```python
from build123d import *

# Parameters (mm, degrees)
F1_DEPTH = 25.4
F2_R     = 3.3782
F3_DEPTH = 25.4
F4_R     = 3.3782
F5_DEPTH = 25.4


with BuildPart() as f1:
    # F0 (on Right) → F1 (new body)
    with BuildSketch(Plane.YZ):
        Polygon((0, 38.1), (0, 0), (38.1, 0), (38.1, 3.175), (3.175, 3.175), (3.175, 38.1), align=None)
    extrude(amount=F1_DEPTH)

    # F2 (on face) → F3 (cut)
    with BuildSketch(Plane.XZ):
        with Locations((12.7, 19.05)):
            Circle(F2_R)
    extrude(amount=-F3_DEPTH, mode=Mode.SUBTRACT)

    # F4 (on face) → F5 (cut)
    with BuildSketch(Plane(origin=(0, 0, 0), x_dir=(1, 0, 0), z_dir=(0, 0, -1))):
        with Locations((12.7, -19.05)):
            Circle(F4_R)
    extrude(amount=-F5_DEPTH, mode=Mode.SUBTRACT)


solid = f1.part
```
Could you check a few things on this model? Use its own coordinates, in mm. A direction names the side the tool comes from. Coordinates: 2 decimals unless noted, no trailing zeros. Order: outer loops, then holes, each group sorted by start corner. A loop starts at its lowest first (then second) coordinate and runs counter-clockwise, first axis right, second up. Notation, with made-up numbers: M 6,65 L 62,65 A29 ccw 62,85 Z; hole C 52.5,60 d1. An arc over 180 degrees is marked long. Use a Markdown table: item, result. Add a question column.
Q1. I'm going to push a flat-ended pin straight in: pin 1 (1 mm diameter, centred on x = 5, z = 19.5, fed in from +Y) (3 decimals). Where does the tip first touch, or does it pass through?
Q2. I want a section at A-A on y = 19.05. List the corners of the cut face in (x, z) for me (3 decimals), then the cut area to 3 significant figures.
Q3. If I drill on L1, parallel to X at y = 19.05, z = 2; L2, parallel to Y at x = 12.7, z = 0.95; L3, parallel to Z at x = 17.5, y = 8 (3 decimals), over which ranges is the centre line in solid material (lowest first)?
Q4. I want a section at B-B on x = 12.7. List the corners of the cut face in (y, z) for me (3 decimals).
Q5. I want a section at D-D on x = 15.25. List the corners of the cut face in (y, z) for me (3 decimals).
Q6. Which directions (+Z, -Z, +X, -X, +Y, -Y) give clear straight access to the entire face, cutting with the end or side of a thin tool? Please do faces 1 (the flat face through (13, 2, 38.1)), 2 (the flat face through (13, 25, 3.175)).
Q7. We'd pull the mould along X, two halves only. Please class faces 3 (the cylindrical face through (12.26, 15.7, 1.57)), 4 (the cylindrical face through (11.97, 1.57, 15.75)), 5 (the flat face through (25.4, 2, 11)), 6 (the flat face through (13, 38.1, 2)): pulls with the +X half, pulls with the -X half, needs draft (parallel to the pull), parting line crosses it, or undercut.
Checked values:
| question | item | result |
|---|---|---|
| 1 | pin 1 | y = 3.175 |
| 2 | outline | M 0,0 L 9.322,0 L 9.322,3.175 L 0,3.175 Z; M 16.078,0 L 25.4,0 L 25.4,3.175 L 16.078,3.175 Z |
| 2 | area | 59.2 mm² |
| 3 | L1 | 0 to 9.32, 16.08 to 25.4 |
| 3 | L2 | 0 to 15.67, 22.43 to 38.1 |
| 3 | L3 | 0 to 3.175 |
| 4 | outline | M 0,0 L 15.672,0 L 15.672,3.175 L 3.175,3.175 L 3.175,15.672 L 0,15.672 Z; M 0,22.428 L 3.175,22.428 L 3.175,38.1 L 0,38.1 Z; M 22.428,0 L 38.1,0 L 38.1,3.175 L 22.428,3.175 Z |
| 5 | outline | M 0,0 L 16.834,0 L 16.834,3.175 L 3.175,3.175 L 3.175,16.834 L 0,16.834 Z; M 0,21.266 L 3.175,21.266 L 3.175,38.1 L 0,38.1 Z; M 21.266,0 L 38.1,0 L 38.1,3.175 L 21.266,3.175 Z |
| 6 | face 1 | +Z, +X, -X, +Y, -Y |
| 6 | face 2 | +Z, +X, -X, +Y |
| 7 | face 3 | undercut |
| 7 | face 4 | undercut |
| 7 | face 5 | pulls with the +X half |
| 7 | face 6 | needs draft |
